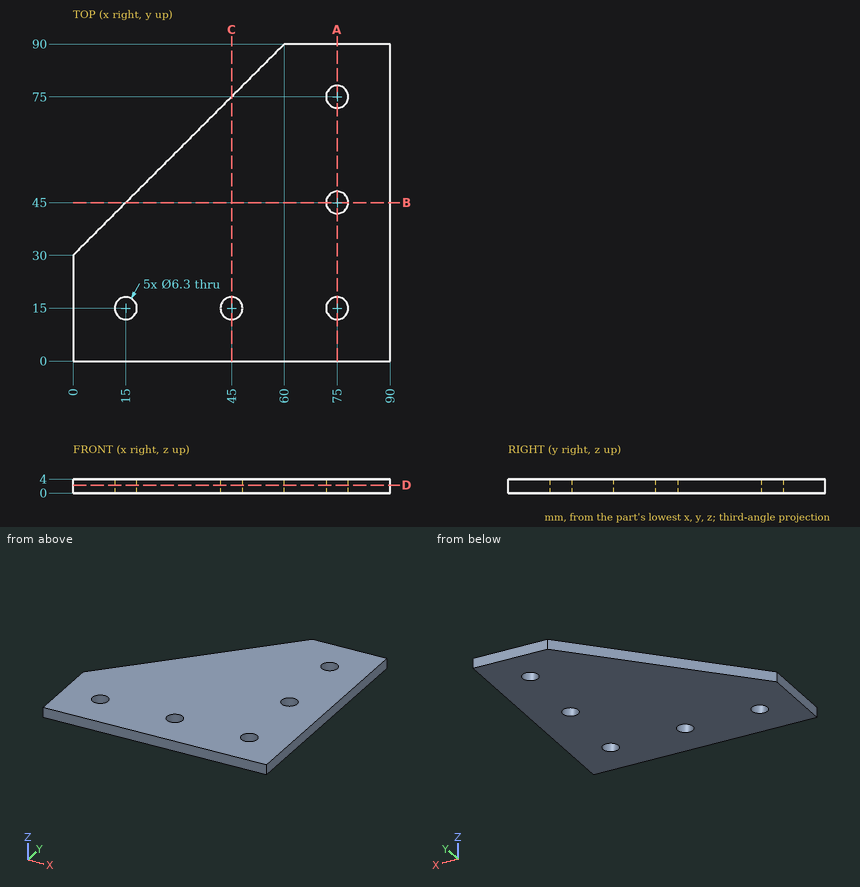
Can you work these out from the drawing? Everything is in mm from the part's minimum corner. Coordinates: 2 decimals unless noted, no trailing zeros. Loops run counter-clockwise (first coordinate to the right, second up) from the corner with the lowest first, then second, coordinate; pieces in that order, holes last. Notation, with made-up numbers: (-6.75, 24.5) - (27.25, 24.5) arc R24 ccw to (27.25, 53.5) - close; hole circle Ø5 at (59, 51). An arc over 180 degrees is marked (long way). Use a Markdown table: item, result.
Item 1: I want a section at A-A on x = 75. Please give me the cut outline in (y, z).
Numbers:
| item | result |
|---|---|
| outline | (0, 0) - (11.85, 0) - (11.85, 4) - (0, 4) - close; (18.15, 0) - (41.85, 0) - (41.85, 4) - (18.15, 4) - close; (48.15, 0) - (71.85, 0) - (71.85, 4) - (48.15, 4) - close; (78.15, 0) - (90, 0) - (90, 4) - (78.15, 4) - close |
Item 2: I want a section at D-D on z = 2.25. Please give me the cut outline in (x, y), and give its area (3 significant figures).
Numbers:
| item | result |
|---|---|
| outline | (0, 0) - (90, 0) - (90, 90) - (60, 90) - (0, 30) - close; hole circle Ø6.3 at (15, 15); hole circle Ø6.3 at (45, 15); hole circle Ø6.3 at (75, 15); hole circle Ø6.3 at (75, 45); hole circle Ø6.3 at (75, 75) |
| area | 6,140 mm2 |
Item 3: If I drill on probe 1 along Y at (x, z) = (75, 1.5); probe 2 along Y at (x, z) = (14, 3.55); probe 3 along X at (y, z) = (75.5, 1.45), over which ranges is the centre line in solid material (lowest first)? Write a range as from..to.
Numbers:
| item | result |
|---|---|
| probe 1 | y = 0..11.85, 18.15..41.85, 48.15..71.85, 78.15..90 |
| probe 2 | y = 0..12.01, 17.99..44 |
| probe 3 | x = 45.5..71.89, 78.11..90 |
Item 4: I want a section at C-C on x = 45. Please give me the cut outline in (y, z), and give its area (3 significant figures).
Numbers:
| item | result |
|---|---|
| outline | (0, 0) - (11.85, 0) - (11.85, 4) - (0, 4) - close; (18.15, 0) - (75, 0) - (75, 4) - (18.15, 4) - close |
| area | 275 mm2 |
Item 5: I want a section at B-B on y = 45. Please give me the cut outline in (x, z).
Numbers:
| item | result |
|---|---|
| outline | (15, 0) - (71.85, 0) - (71.85, 4) - (15, 4) - close; (78.15, 0) - (90, 0) - (90, 4) - (78.15, 4) - close |
